Autodesk Inventor part; units mm, degrees
ref_plane "YZ Plane" through (0, 0, 0) normal (1, 0, 0) x (0, 1, 0)
ref_plane "XZ Plane" through (0, 0, 0) normal (0, 1, 0) x (-1, 0, 0)
ref_plane "XY Plane" through (0, 0, 0) normal (0, 0, 1) x (1, 0, 0)
sketch "スケッチ1" plane through (0, 0, 0) normal (0, 0, 1) x (1, 0, 0)
  line L0 (0, 3.1754) -> (2.75, 1.5877)
  line L1 (2.75, 1.5877) -> (2.75, -1.5877)
  line L2 (2.75, -1.5877) -> (0, -3.1754)
  line L3 (0, -3.1754) -> (-2.75, -1.5877)
  line L4 (-2.75, -1.5877) -> (-2.75, 1.5877)
  line L5 (-2.75, 1.5877) -> (0, 3.1754)
  point P0 (0, 0)
  point P1 (0, 0)
  dimension "d0" = 5.5
extrude "押し出し1" add sketch "スケッチ1" along normal blind 100
sketch "スケッチ2" plane through (0, 0, 100) normal (0, 0, 1) x (1, 0, 0)
  circle A0 centre (0, 0) radius 1.5
  dimension "d3" = 3
extrude "押し出し2" add sketch "スケッチ2" along normal blind 6
thread "ねじ1"
sketch "スケッチ3" plane through (0, 0, 0) normal (0, 0, -1) x (-1, 0, 0)
  point P0 (0, 0)
hole "穴1" at (0, 0, 0) direction (0, 0, 1) diameter 2.459 depth 8.8 tip angle 118
properties part number "ステンレススペーサー（六角）_BSU-3100" material "ステンレス鋼"
Verification items for the finished model (mm, model axes). A direction names the side the tool comes from. Give positions to 0.01 mm unless a question says otherwise; leave off trailing zeros. Write each loop counter-clockwise with the first axis right and the second up, starting at its lowest first coordinate (ties: lowest second). Pieces come first, ordered by that corner, then holes. Notation, with made-up numbers: M -30,55 L -4,55 A15 ccw -4,68 Z; hole C -16,50 d3. An arc over 180 degrees is marked long. Put each result on its own line as item: value. Start each with the question number.
1. Set-up check for faces 4 (the face through (0.748, -0.976, 4.462)), 5 (the face through (-1.5, -0.07, 102.96)), 6 (the face through (0, -1.4, 0)): record each of +Z, -Z, +X, -X, +Y, -Y from which the full face is reachable in a straight line by a thin tool's end or side.
2. Section check A-A (z = 31.5). Record the cut outline in (x, y).
3. Scan lines: line 1 along Y through (x, z) = (0, 3.25); line 2 along X through (y, z) = (0, 6.75); line 3 along Z through (x, y) = (-2.35, -1.5). Record each from-to range of solid material in increasing order. Write a range as [from, to].
4. Go/stop test with flat-tipped pins: pin 1 Ø3 at (x, z) = (2, 46) entering from -Y; pin 2 Ø3 at (x, z) = (0.5, 25.5) entering from +Y; pin 3 Ø2 at (x, y) = (-1.5, 2.5) entering from +Z. Record where each tip stops, or that it passes through.
5. Draft check along Y on faces 1 (the face through (0, 0, 106)), 2 (the face through (0.064, 0.204, 9.41)), 3 (the face through (1.394, -2.37, 49.3)). Enter one of: +Y half, -Y half, draft (parallel to the pull), parting line (faces both ways), or undercut.
Answer list:
1. face 4: -Z
1. face 5: +Z
1. face 6: -Z, +X, -X, +Y, -Y
2. outline: M -2.75,-1.59 L 0,-3.18 L 2.75,-1.59 L 2.75,1.59 L 0,3.18 L -2.75,1.59 Z
3. line 1: [-3.18, -1.23], [1.23, 3.18]
3. line 2: [-2.75, -1.23], [1.23, 2.75]
3. line 3: [0, 100]
4. pin 1: y = -2.89
4. pin 2: y = 3.18
4. pin 3: z = 100
5. face 1: draft
5. face 2: undercut
5. face 3: -Y half
